The listing builds one solid part. Answer for the finished solid, in the listing's coordinates (mm). A direction names the side the tool comes from. Give positions to 0.01 mm unless a question says otherwise; leave off trailing zeros. Order: outer loops, then holes, each group sorted by start corner. A loop starts at its lowest first (then second) coordinate and runs counter-clockwise, first axis right, second up. Notation, with made-up numbers: (57.25, 32.25) - (85.25, 32.25) arc R9 cw to (85.25, 38.25) - close; hole circle Ø7 at (9, -2). An arc over 180 degrees is marked (long way). Use a Markdown table: item, result. Add a question column.
1) For faces 1 (the face through (-4.101, -31.232, 264.248)), 2 (the face through (31, 0, 55)), determine the directions among +Z, -Z, +X, -X, +Y, -Y from which every point of the face is accessible in a straight line to the end or side of a thin tool.
2) Find section A-A, the plane y = -17. Determine the outline of the cut face in (x, z).
3) Find section C-C, the plane x = -12.5. Determine the outline of the cut face in (y, z).
4) Flat-ended cylindrical pins translate along their axes: pin 1 (2 mm diameter, centred on x = -2, z = 310, fed in from -Y); pin 2 (1 mm diameter, centred on x = 2.5, z = 326, fed in from +Y); pin 3 (2 mm diameter, centred on y = -22, z = 193.5, fed in from +X); pin 4 (1.6 mm diameter, centred on y = 0, z = 40, fed in from -X). Find the tip coordinate at first contact, or state that the pin passes through.
5) Find section D-D, the plane z = 66.5. Determine the outline of the cut face in (x, y), plus the area to 3 significant figures.
6) Find section B-B, the plane z = 174.5. Determine the outline of the cut face in (x, y).
7) Straight lines are drawn through the part: line 1 (X direction, y = 0, z = 332); line 2 (Z direction, x = 29, y = 0); line 3 (Y direction, x = 28.55, z = 80). For each, find the intervals that lie inside material, in ascending order.
Autodesk Inventor part; units mm, degrees
ref_plane "Work Plane6" through (31.5, 0, 536) normal (1, 0, 0) x (0, 1, 0)
ref_plane "Work Plane7" through (31, 0, 0) normal (1, 0, 0) x (0, 1, 0)
ref_plane "Work Plane8" through (-0.7293, 31.4916, 0) normal (0, -0.3156, -0.9489) x (-1, 0, 0)
sketch "Sketch1" plane through (0, 0, 0) normal (0, 0, 1) x (1, 0, 0)
  circle A0 centre (0, 0) radius 31.5
  circle A1 centre (0, 0) radius 27.9
  dimension "d0" = 63
  dimension "d2" = 3.6
extrude "tube" add sketch "Sketch1" along normal blind 536
sketch "Sketch15" plane through (0, 0, 536) normal (0, 0, 1) x (1, 0, 0)
  circle A0 centre (0, 0) radius 27.9
  circle A1 centre (0, 0) radius 31.5
  point P0 (31.5, 0)
ref_plane "Work Plane6" through (31.5, 0, 536) normal (1, 0, 0) x (0, 1, 0)
ref_plane "Work Plane7" through (31, 0, 0) normal (1, 0, 0) x (0, 1, 0)
sketch "Sketch19" plane through (31, 0, 0) normal (1, 0, 0) x (0, 1, 0)
  line L0 (-10, 0) -> (10, 0)
  line L1 (10, 0) -> (10, 100)
  line L2 (10, 100) -> (-10, 100)
  line L3 (-10, 100) -> (-10, 0)
  point P0 (0, 0)
  point P1 (0, 0)
  dimension "d67" = 20
  dimension "d68" = 100
extrude "flatFaceYellow" cut sketch "Sketch19" along normal blind 25.4
sketch "Sketch21" plane through (0, 0, 0) normal (0, 0, -1) x (-1, 0, 0)
  line L0 (-31, 5.5902) -> (-31, -5.5902)
  arc A0 (-31, -5.5902) -> (-31, 5.5902) centre (0, 0) ccw
  circle A1 centre (0, 0) radius 27.9
  line L1 (0.7293, 31.4916) -> (30.8537, 31.4916) construction
ref_plane "Work Plane8" through (-0.7293, 31.4916, 0) normal (0, -0.3156, -0.9489) x (-1, 0, 0)
sketch "Sketch22" plane through (-0.7293, 31.4916, 0) normal (0, -0.3156, -0.9489) x (-1, 0, 0)
  line L0 (-34.8075, -84.5558) -> (31.7452, -84.5558)
  line L1 (31.7452, -84.5558) -> (31.7452, 8.8585)
  line L2 (31.7452, 8.8585) -> (-34.8075, 8.8585)
  line L3 (-34.8075, 8.8585) -> (-34.8075, -84.5558)
  point P0 (-0.7293, -29.8816)
extrude "angledEnd" cut sketch "Sketch22" along normal blind 25.4
sketch "Sketch23" plane through (31, 0, 0) normal (1, 0, 0) x (0, 0, -1)
  line L0 (-12.3354, -5.5902) -> (-100, -5.5902)
  circle A0 centre (-80, 0) radius 3.2074
  circle A1 centre (-40, 0) radius 3.2074
  point P0 (0, 0)
  dimension "d89" = 80
  dimension "d92" = 40
hole "Hole3" at (31, 0, 80) at (31, 0, 40) direction (-1, 0, 0) diameter 2 end through all
properties part number "sparVert_B" material "PVC-Piping"
The answers:
| question | item | result |
|---|---|---|
| 1 | face 1 | +Z, -Z |
| 1 | face 2 | -Z, +X, +Y, -Y |
| 2 | outline | (-26.52, 16.13) - (-22.12, 16.13) - (-22.12, 536) - (-26.52, 536) - close; (22.12, 16.13) - (26.52, 16.13) - (26.52, 536) - (22.12, 536) - close |
| 3 | outline | (-28.91, 20.09) - (-24.94, 18.77) - (-24.94, 536) - (-28.91, 536) - close; (24.94, 2.18) - (28.91, 0.86) - (28.91, 536) - (24.94, 536) - close |
| 4 | pin 1 | y = -31.48 |
| 4 | pin 2 | y = 31.44 |
| 4 | pin 3 | x = 23.48 |
| 4 | pin 4 | through |
| 5 | outline | (31, -5.59) - (31, 5.59) arc R31.5 ccw (long way) to start; hole circle Ø55.8 at (0, 0) |
| 5 | area | 668 mm2 |
| 6 | outline | circle Ø63 at (0, 0); hole circle Ø55.8 at (0, 0) |
| 7 | line 1 | -31.5 to -27.9, 27.9 to 31.5 |
| 7 | line 2 | 10.48 to 39, 41 to 79, 81 to 536 |
| 7 | line 3 | -13.31 to -1, 1 to 13.31 |
